Check sheet for the modelled part. Datum: model origin and axes. Units: mm. A direction names the side the tool comes from. Give positions to 0.01 mm unless a question says otherwise; leave off trailing zeros. Order: outer loops, then holes, each group sorted by start corner. A loop starts at its lowest first (then second) coordinate and runs counter-clockwise, first axis right, second up. Notation, with made-up numbers: (33.5, -35) - (61.5, -35) arc R15 cw to (61.5, -28) - close; hole circle Ø10 at (6.5, 13). An arc over 180 degrees is marked (long way). Answer in a Markdown table with one row per item.
from build123d import *

# Parameters (mm, degrees)
SKETCH1_R           = 16.764
BOSS_EXTRUDE1_DEPTH = 300
SKETCH2_R           = 16.764
BOSS_EXTRUDE2_DEPTH = 50
SHELL1_START        = 3
SHELL1_OUTLINE_R    = 13.764
SHELL1_DEPTH        = 297
SHELL1_START_2      = -1e-07
SHELL1_2_OUTLINE_R  = 13.764
SHELL1_2_DEPTH      = 47.0000001
SKETCH3_R           = 12.7
CUT_EXTRUDE1_DEPTH  = 20
SKETCH4_R           = 13.764
CUT_EXTRUDE2_DEPTH  = 302.645539824


with BuildPart() as part:
    # Sketch1 → Boss-Extrude1 (new body)
    with BuildSketch(Plane(origin=(0, 0, 0), x_dir=(1, 0, 0), z_dir=(0, 1, 0))):
        with Locations(Location((0, 0, 0), (0, 0, 270))):
            Circle(SKETCH1_R)
    extrude(amount=BOSS_EXTRUDE1_DEPTH)

    # Sketch2 → Boss-Extrude2 (add)
    with BuildSketch(Plane.XY):
        with Locations((0, 100)):
            Circle(SKETCH2_R)
    extrude(amount=BOSS_EXTRUDE2_DEPTH)

    # Shell1: read off the stored shape, not the designer's step
    # Shell1 outline → Shell1 (cut)
    with BuildSketch(Plane(origin=(0, 0, 0), x_dir=(1, 0, 0), z_dir=(0, 1, 0)).offset(SHELL1_START)):
        Circle(SHELL1_OUTLINE_R)
    extrude(amount=SHELL1_DEPTH, mode=Mode.SUBTRACT)

    # Shell1 2 outline → Shell1 2 (cut)
    with BuildSketch(Plane.XY.offset(SHELL1_START_2)):
        with Locations((0, 100)):
            Circle(SHELL1_2_OUTLINE_R)
    extrude(amount=SHELL1_2_DEPTH, mode=Mode.SUBTRACT)

    # Sketch3 → Cut-Extrude1 (cut)
    with BuildSketch(Plane.XY.offset(50)):
        with Locations((0, 100)):
            Circle(SKETCH3_R)
    extrude(amount=-CUT_EXTRUDE1_DEPTH, mode=Mode.SUBTRACT)

    # Sketch4 → Cut-Extrude2 (cut, through all)
    with BuildSketch(Plane(origin=(0, 3, 0), x_dir=(1, 0, 0), z_dir=(0, 1, 0))):
        with Locations(Location((0, 0, 0), (0, 0, 270))):
            Circle(SKETCH4_R)
    extrude(amount=-CUT_EXTRUDE2_DEPTH, mode=Mode.SUBTRACT)


solid = part.part
(1) Mould release check, pull along X, two halves, no side actions. Record for faces 1 (the cylindrical face through (0.737, 147.9, -16.748)), 2 (the flat face through (-12.5, 103.8, 50)), 3 (the cylindrical face through (13.13, 104.13, 28.39)): pulls with the +X half, pulls with the -X half, needs draft (parallel to the pull), parting line crosses it, or undercut.
Geometry says:
| item | result |
|---|---|
| face 1 | parting line crosses it |
| face 2 | needs draft |
| face 3 | undercut |
(2) Cross-section at A-A, the plane x = 0. Record the cut outline in (y, z), then the cut area to 3 significant figures.
Geometry says:
| item | result |
|---|---|
| outline | (0, -16.76) - (300, -16.76) - (300, -13.76) - (0, -13.76) - close; (0, 13.76) - (86.24, 13.76) - (86.24, 47) - (87.3, 47) - (87.3, 50) - (83.24, 50) - (83.24, 16.76) - (0, 16.76) - close; (112.7, 47) - (113.76, 47) - (113.76, 13.76) - (300, 13.76) - (300, 16.76) - (116.76, 16.76) - (116.76, 50) - (112.7, 50) - close |
| area | 1,920 mm² |
(3) Cross-section at C-C, the plane y = 228. Record the cut outline in (x, z).
Geometry says:
| item | result |
|---|---|
| outline | circle Ø33.53 at (0, 0); hole circle Ø27.53 at (0, 0) |
(4) Cross-section at B-B, the plane y = 100. Record the cut outline in (x, z).
Geometry says:
| item | result |
|---|---|
| outline | (-16.76, 0) arc R16.76 ccw to (16.76, 0) - (16.76, 50) - (12.7, 50) - (12.7, 47) - (13.76, 47) - (13.76, 0) arc R13.76 cw to (-13.76, 0) - (-13.76, 47) - (-12.7, 47) - (-12.7, 50) - (-16.76, 50) - close |
(5) Thickness scan on L1, parallel to X at y = 100, z = 37; L2, parallel to Y at x = 0, z = 29; L3, parallel to Z at x = -3.5, y = 150.5. Record the ranges inside material, lowest first.
Geometry says:
| item | result |
|---|---|
| L1 | -16.76 to -13.76, 13.76 to 16.76 |
| L2 | 83.24 to 86.24, 113.76 to 116.76 |
| L3 | -16.39 to -13.31, 13.31 to 16.39 |
(6) Access from +Z, -Z, +X, -X, +Y, -Y to the whole of each face (thin tool, end or side, straight path). Record for faces 4 (the cylindrical face through (-2.75, 87.6, 48.52)), 5 (the flat face through (9.1, 90.9, 47)), 6 (the flat face through (14, 0, -1)).
Geometry says:
| item | result |
|---|---|
| face 4 | +Z |
| face 5 | none |
| face 6 | +Z, -Z, +X, -X, -Y |
(7) Gauge pin test, flat ends, axial feed: P1, Ø3, axis at y = 103, z = -5, coming from the +X side; P2, Ø8, axis at x = -8.5, y = 221.5, coming from the -Z side; P3, Ø4, axis at y = 82.5, z = 31.5, coming from the -X side. Record the tip position at first contact, or that the pin passes through.
Geometry says:
| item | result |
|---|---|
| P1 | x = 16.39 |
| P2 | z = -16.15 |
| P3 | x = -6.39 |
